from build123d import *

# Parameters (mm, degrees)
SKETCH1_W           = 76
SKETCH1_H           = 56
BOSS_EXTRUDE1_DEPTH = 3.5
SKETCH2_R           = 4.5
SKETCH2_W           = 22
SKETCH2_H           = 16
CUT_EXTRUDE1_DEPTH  = 3.5


with BuildPart() as part:
    # Sketch1 → Boss-Extrude1 (new body)
    with BuildSketch(Plane(origin=(0, 0, 0), x_dir=(1, 0, 0), z_dir=(0, 1, 0))):
        Rectangle(SKETCH1_W, SKETCH1_H)
    extrude(amount=BOSS_EXTRUDE1_DEPTH)

    # Sketch2 → Cut-Extrude1 (cut)
    with BuildSketch(Plane.XZ):
        with Locations((0, -30)):
            Circle(SKETCH2_R)
        with Locations((0, 30)):
            Circle(SKETCH2_R)
        Rectangle(SKETCH2_W, SKETCH2_H)
    extrude(amount=-CUT_EXTRUDE1_DEPTH, mode=Mode.SUBTRACT)


solid = part.part
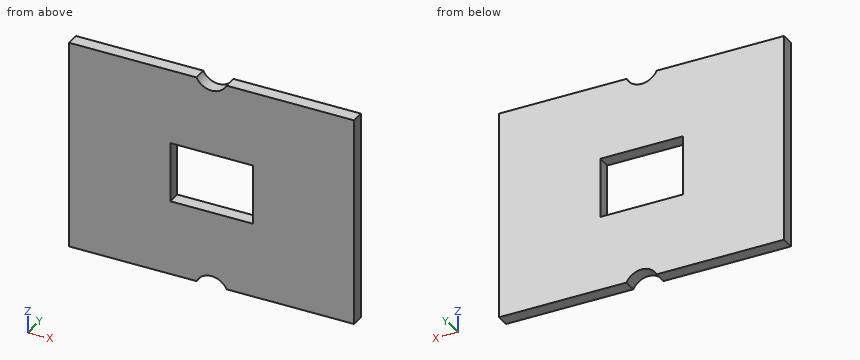
For this review, take the finished solid that the model builds, in its own axes (mm). Round coordinates to 2 decimals unless told otherwise and drop trailing zeros. Order: outer loops, then holes, each group sorted by start corner. A loop starts at its lowest first (then second) coordinate and runs counter-clockwise, first axis right, second up. Notation, with made-up numbers: (62, 77) -> (117, 77) arc R13 cw to (117, 96) -> close; hole circle Ø5 at (9.5, -13). An arc over 180 degrees is marked (long way). Write item = value, one per line. Start each with the question number.
1) Take a section at A-A on x = -6. State the section outline as (y, z) points, plus the area to 3 significant figures.
2) Take a section at B-B on y = 0.95. State the section outline as (x, z) points, plus the area to 3 significant figures.
3) To check wall thickness, follow line 1 (X direction, y = 0.65, z = -0.5); line 2 (Z direction, x = -7, y = 0.6); line 3 (Z direction, x = -2.5, y = 0.25). State the ranges of each line that lie inside material, in increasing order. Write a range as from..to.
Verdict:
q1.outline = (0, -28) -> (3.5, -28) -> (3.5, -8) -> (0, -8) -> close; (0, 8) -> (3.5, 8) -> (3.5, 28) -> (0, 28) -> close
q1.area = 140 mm2
q2.outline = (-38, -28) -> (-4.03, -28) arc R4.5 cw to (4.03, -28) -> (38, -28) -> (38, 28) -> (4.03, 28) arc R4.5 cw to (-4.03, 28) -> (-38, 28) -> close; hole (-11, -8) -> (11, -8) -> (11, 8) -> (-11, 8) -> close
q2.area = 3,880 mm2
q3.line_1 = -38..-11, 11..38
q3.line_2 = -28..-8, 8..28
q3.line_3 = -26.26..-8, 8..26.26
